Answer from the drawing. Dimensions are ordinates in mm from the lowest x, y and z of the part. A direction names the side the tool comes from. Give positions to 0.01 mm unless a question says otherwise; leave off trailing zeros. Loops run counter-clockwise (first coordinate to the right, second up) from the corner with the lowest first, then second, coordinate; pieces in that order, holes last.
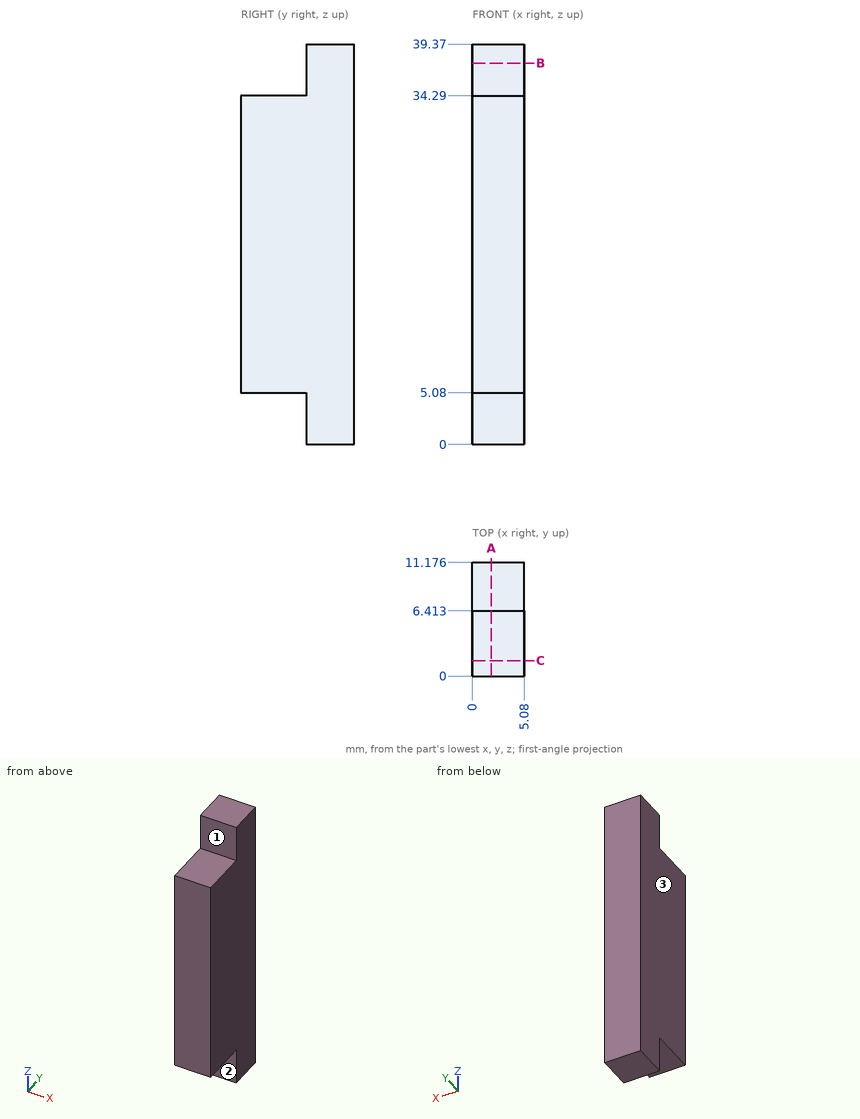
Item 1: Find section C-C, the plane y = 1.5. Write down the section's boundary in (x, z).
Item 2: Find section A-A, the plane x = 1.85. Write down the section's boundary in (y, z) (1 decimal), plus the area to 3 significant figures.
Item 3: A flat-ended cylindrical pin translates along its axis: pin 1 Ø1.5 at (x, z) = (3, 36.5) entering from -Y. Find the tip coordinate at first contact, or state that the pin passes through.
Item 4: For the marked faces 1, 2 and 3, determine the directions among +Z, -Z, +X, -X, +Y, -Y from which every point of the face is accessible in a straight line to the end or side of a thin tool.
Item 5: Consider line 1 (Z direction, x = 3.35, y = 6.25); line 2 (Y direction, x = 2.7, z = 4) (1 decimal). Determine where each line is inside the solid, lowest interval first.
Item 6: Find section B-B, the plane z = 37.5. Write down the section's boundary in (x, y) (1 decimal), plus the area to 3 significant figures.
Ans:
1. outline: (0, 5.08) - (5.08, 5.08) - (5.08, 34.29) - (0, 34.29) - close
2. outline: (0, 5.1) - (6.4, 5.1) - (6.4, 0) - (11.2, 0) - (11.2, 39.4) - (6.4, 39.4) - (6.4, 34.3) - (0, 34.3) - close
2. area: 375 mm2
3. pin 1: stops at y = 6.41
4. face 1: +Z, +X, -X, -Y
4. face 2: -Z, +X, -X, -Y
4. face 3: +Z, -Z, -X, +Y, -Y
5. line 1: z = 5.08 to 34.29
5. line 2: y = 6.4 to 11.2
6. outline: (0, 6.4) - (5.1, 6.4) - (5.1, 11.2) - (0, 11.2) - close
6. area: 24.2 mm2
